Here's how the part is built. I have some questions about the finished solid (model axes, mm). A direction names the side the tool comes from. Round coordinates to 2 decimals unless told otherwise and drop trailing zeros. Loops run counter-clockwise (first coordinate to the right, second up) from the corner with the lowest first, then second, coordinate; pieces in that order, holes last. Notation, with made-up numbers: M 41.5,-1 L 64.5,-1 A15 cw 64.5,18 Z; hole C -22,31.5 d8. An arc over 180 degrees is marked long. Write each question's results on one line, items separated by ' | '. Start each with the question number.
```python
from build123d import *

# Parameters (mm, degrees)
SCHIZZO1_W                   = 94.84
SCHIZZO1_H                   = 59.15
ESTRUSIONE_ESTRUSIONE1_DEPTH = 0.8
SCHIZZO2_R                   = 1.5
TAGLIO_ESTRUSIONE1_DEPTH     = 56.909722097
SCHIZZO3_R                   = 0.445
TAGLIO_ESTRUSIONE2_DEPTH     = 56.909722097
ESTRUSIONE_ESTRUSIONE2_START = 0.01
SCHIZZO4_R                   = 2
SCHIZZO4_R_2                 = 1.5
SCHIZZO4_R_3                 = 0.745
SCHIZZO4_R_4                 = 0.445
ESTRUSIONE_ESTRUSIONE2_DEPTH = 0.01
SCHIZZO5_W                   = 85
SCHIZZO5_H                   = 55.26
ESTRUSIONE_ESTRUSIONE3_DEPTH = 2.4
SCHIZZO7_W                   = 73.44
SCHIZZO7_H                   = 48.96
TAGLIO_ESTRUSIONE3_DEPTH     = 0.5


with BuildPart() as part:
    # Schizzo1 → Estrusione-Estrusione1 (new, symmetric)
    with BuildSketch(Plane(origin=(0, 0, 0), x_dir=(1, 0, 0), z_dir=(0, 1, 0))):
        Rectangle(SCHIZZO1_W, SCHIZZO1_H)
    extrude(amount=ESTRUSIONE_ESTRUSIONE1_DEPTH, both=True)

    # Schizzo2 → Taglio-Estrusione1 (cut, through all)
    with BuildSketch(Plane(origin=(0, 0.8, 0), x_dir=(1, 0, 0), z_dir=(0, 1, 0))):
        with Locations(Location((-45.26, 24, 0), (0, 0, 270))):
            Circle(SCHIZZO2_R)
        with Locations(Location((44.75, 24, 0), (0, 0, 270))):
            Circle(SCHIZZO2_R)
        with Locations(Location((44.75, -24, 0), (0, 0, 270))):
            Circle(SCHIZZO2_R)
        with Locations(Location((-45.26, -24, 0), (0, 0, 270))):
            Circle(SCHIZZO2_R)
    extrude(amount=-TAGLIO_ESTRUSIONE1_DEPTH, mode=Mode.SUBTRACT)

    # Schizzo3 → Taglio-Estrusione2 (cut, through all)
    with BuildSketch(Plane(origin=(0, 0.8, 0), x_dir=(1, 0, 0), z_dir=(0, 1, 0))):
        with Locations(Location((-45.67, 0, 0), (0, 0, 270))):
            Circle(SCHIZZO3_R)
        with Locations(Location((-45.67, -2.54, 0), (0, 0, 270))):
            Circle(SCHIZZO3_R)
        with Locations(Location((-45.67, -5.08, 0), (0, 0, 270))):
            Circle(SCHIZZO3_R)
        with Locations(Location((-45.67, -7.62, 0), (0, 0, 270))):
            Circle(SCHIZZO3_R)
        with Locations(Location((-45.67, -10.16, 0), (0, 0, 270))):
            Circle(SCHIZZO3_R)
        with Locations(Location((-45.67, 2.54, 0), (0, 0, 270))):
            Circle(SCHIZZO3_R)
        with Locations(Location((-45.67, 5.08, 0), (0, 0, 270))):
            Circle(SCHIZZO3_R)
        with Locations(Location((-45.67, 7.62, 0), (0, 0, 270))):
            Circle(SCHIZZO3_R)
        with Locations(Location((-45.67, 10.16, 0), (0, 0, 270))):
            Circle(SCHIZZO3_R)
    extrude(amount=-TAGLIO_ESTRUSIONE2_DEPTH, mode=Mode.SUBTRACT)

    # Schizzo4 → Estrusione-Estrusione2 (add)
    # profile 1 of 13: a face of its own
    with BuildSketch(Plane(origin=(0, 0.8, 0), x_dir=(1, 0, 0), z_dir=(0, 1, 0)).offset(ESTRUSIONE_ESTRUSIONE2_START)):
        with Locations(Location((44.75, 24, 0), (0, 0, 90))):
            Circle(SCHIZZO4_R)
        with Locations(Location((44.75, 24, 0), (0, 0, 270))):
            Circle(SCHIZZO4_R_2, mode=Mode.SUBTRACT)
    # profile 2 of 13: a face of its own
    with BuildSketch(Plane(origin=(0, 0.8, 0), x_dir=(1, 0, 0), z_dir=(0, 1, 0)).offset(ESTRUSIONE_ESTRUSIONE2_START)):
        with Locations(Location((-45.26, 24, 0), (0, 0, 90))):
            Circle(SCHIZZO4_R)
        with Locations(Location((-45.26, 24, 0), (0, 0, 270))):
            Circle(SCHIZZO4_R_2, mode=Mode.SUBTRACT)
    # profile 3 of 13: a face of its own
    with BuildSketch(Plane(origin=(0, 0.8, 0), x_dir=(1, 0, 0), z_dir=(0, 1, 0)).offset(ESTRUSIONE_ESTRUSIONE2_START)):
        with Locations(Location((-45.26, -24, 0), (0, 0, 90))):
            Circle(SCHIZZO4_R)
        with Locations(Location((-45.26, -24, 0), (0, 0, 270))):
            Circle(SCHIZZO4_R_2, mode=Mode.SUBTRACT)
    # profile 4 of 13: a face of its own
    with BuildSketch(Plane(origin=(0, 0.8, 0), x_dir=(1, 0, 0), z_dir=(0, 1, 0)).offset(ESTRUSIONE_ESTRUSIONE2_START)):
        with Locations(Location((44.75, -24, 0), (0, 0, 90))):
            Circle(SCHIZZO4_R)
        with Locations(Location((44.75, -24, 0), (0, 0, 270))):
            Circle(SCHIZZO4_R_2, mode=Mode.SUBTRACT)
    # profile 5 of 13: a face of its own
    with BuildSketch(Plane(origin=(0, 0.8, 0), x_dir=(1, 0, 0), z_dir=(0, 1, 0)).offset(ESTRUSIONE_ESTRUSIONE2_START)):
        with Locations(Location((-45.67, 10.16, 0), (0, 0, 90))):
            Circle(SCHIZZO4_R_3)
        with Locations(Location((-45.67, 10.16, 0), (0, 0, 270))):
            Circle(SCHIZZO4_R_4, mode=Mode.SUBTRACT)
    # profile 6 of 13: a face of its own
    with BuildSketch(Plane(origin=(0, 0.8, 0), x_dir=(1, 0, 0), z_dir=(0, 1, 0)).offset(ESTRUSIONE_ESTRUSIONE2_START)):
        with Locations(Location((-45.67, 7.62, 0), (0, 0, 90))):
            Circle(SCHIZZO4_R_3)
        with Locations(Location((-45.67, 7.62, 0), (0, 0, 270))):
            Circle(SCHIZZO4_R_4, mode=Mode.SUBTRACT)
    # profile 7 of 13: a face of its own
    with BuildSketch(Plane(origin=(0, 0.8, 0), x_dir=(1, 0, 0), z_dir=(0, 1, 0)).offset(ESTRUSIONE_ESTRUSIONE2_START)):
        with Locations(Location((-45.67, 5.08, 0), (0, 0, 90))):
            Circle(SCHIZZO4_R_3)
        with Locations(Location((-45.67, 5.08, 0), (0, 0, 270))):
            Circle(SCHIZZO4_R_4, mode=Mode.SUBTRACT)
    # profile 8 of 13: a face of its own
    with BuildSketch(Plane(origin=(0, 0.8, 0), x_dir=(1, 0, 0), z_dir=(0, 1, 0)).offset(ESTRUSIONE_ESTRUSIONE2_START)):
        with Locations(Location((-45.67, 2.54, 0), (0, 0, 90))):
            Circle(SCHIZZO4_R_3)
        with Locations(Location((-45.67, 2.54, 0), (0, 0, 270))):
            Circle(SCHIZZO4_R_4, mode=Mode.SUBTRACT)
    # profile 9 of 13: a face of its own
    with BuildSketch(Plane(origin=(0, 0.8, 0), x_dir=(1, 0, 0), z_dir=(0, 1, 0)).offset(ESTRUSIONE_ESTRUSIONE2_START)):
        with Locations(Location((-45.67, 0, 0), (0, 0, 90))):
            Circle(SCHIZZO4_R_3)
        with Locations(Location((-45.67, 0, 0), (0, 0, 270))):
            Circle(SCHIZZO4_R_4, mode=Mode.SUBTRACT)
    # profile 10 of 13: a face of its own
    with BuildSketch(Plane(origin=(0, 0.8, 0), x_dir=(1, 0, 0), z_dir=(0, 1, 0)).offset(ESTRUSIONE_ESTRUSIONE2_START)):
        with Locations(Location((-45.67, -2.54, 0), (0, 0, 90))):
            Circle(SCHIZZO4_R_3)
        with Locations(Location((-45.67, -2.54, 0), (0, 0, 270))):
            Circle(SCHIZZO4_R_4, mode=Mode.SUBTRACT)
    # profile 11 of 13: a face of its own
    with BuildSketch(Plane(origin=(0, 0.8, 0), x_dir=(1, 0, 0), z_dir=(0, 1, 0)).offset(ESTRUSIONE_ESTRUSIONE2_START)):
        with Locations(Location((-45.67, -5.08, 0), (0, 0, 90))):
            Circle(SCHIZZO4_R_3)
        with Locations(Location((-45.67, -5.08, 0), (0, 0, 270))):
            Circle(SCHIZZO4_R_4, mode=Mode.SUBTRACT)
    # profile 12 of 13: a face of its own
    with BuildSketch(Plane(origin=(0, 0.8, 0), x_dir=(1, 0, 0), z_dir=(0, 1, 0)).offset(ESTRUSIONE_ESTRUSIONE2_START)):
        with Locations(Location((-45.67, -7.62, 0), (0, 0, 90))):
            Circle(SCHIZZO4_R_3)
        with Locations(Location((-45.67, -7.62, 0), (0, 0, 270))):
            Circle(SCHIZZO4_R_4, mode=Mode.SUBTRACT)
    # profile 13 of 13: a face of its own
    with BuildSketch(Plane(origin=(0, 0.8, 0), x_dir=(1, 0, 0), z_dir=(0, 1, 0)).offset(ESTRUSIONE_ESTRUSIONE2_START)):
        with Locations(Location((-45.67, -10.16, 0), (0, 0, 90))):
            Circle(SCHIZZO4_R_3)
        with Locations(Location((-45.67, -10.16, 0), (0, 0, 270))):
            Circle(SCHIZZO4_R_4, mode=Mode.SUBTRACT)
    estrusione_estrusione2 = extrude(amount=-ESTRUSIONE_ESTRUSIONE2_DEPTH)

    # Specchia1: Estrusione-Estrusione2 across plane
    add(estrusione_estrusione2.mirror(Plane.ZX))

    # Schizzo5 → Estrusione-Estrusione3 (add)
    with BuildSketch(Plane(origin=(0, 0.8, 0), x_dir=(1, 0, 0), z_dir=(0, 1, 0))):
        with Locations((-0.02, 0)):
            Rectangle(SCHIZZO5_W, SCHIZZO5_H)
    extrude(amount=ESTRUSIONE_ESTRUSIONE3_DEPTH)

    # Schizzo7 → Taglio-Estrusione3 (cut)
    with BuildSketch(Plane(origin=(0, 3.2, 0), x_dir=(1, 0, 0), z_dir=(0, 1, 0))):
        with Locations((-3.05, 0)):
            Rectangle(SCHIZZO7_W, SCHIZZO7_H)
    extrude(amount=-TAGLIO_ESTRUSIONE3_DEPTH, mode=Mode.SUBTRACT)


solid = part.part
```
Item 1: Which directions (+Z, -Z, +X, -X, +Y, -Y) give clear straight access to the entire face, cutting with the end or side of a thin tool? Please do faces 4 (the face through (-1, 2, 27.63)), 5 (the face through (-1, -0.8, 0)), 6 (the face through (43, 0.81, -24)), 7 (the face through (-47, 0.81, -24)).
Item 2: If we mould it in two halves opening along X, with no side actions, what happens to faces 1 (the face through (42.48, 2, 0)), 2 (the face through (-47, -0.81, -24)), 3 (the face through (-4, 2.7, 0))? For each: released by +X, released by -X, zero draft, split by the parting line, or undercut.
Item 3: If we section it at C-C on z = 20.5: Please give me the cut outline in (x, y).
Item 4: If we section it at D-D on y = 1.9: Please give me the cut outline in (x, z).
Item 5: I need wall thicknesses on L1, parallel to X at y = 0, z = 24; L2, parallel to X at y = 2.9, z = 7; L3, parallel to Z at x = 8, y = 1.95. Which ranges of each line are inside material? Lowest first, please.
Item 6: I'm going to push flat-ended pins straight in: pin 1 (3 mm diameter, centred on x = -46, z = -23, fed in from +Y); pin 2 (2.5 mm diameter, centred on x = -45.26, z = 24, fed in from +Y); pin 3 (10 mm diameter, centred on x = 7.5, z = 11.5, fed in from -Y); pin 4 (0.6 mm diameter, centred on x = 13.5, y = 3, fed in from +Z). Where does each tip first touch, or does it pass through?
Item 7: If we section it at A-A on x = 44.75: Please give me the cut outline in (y, z) (3 decimals), and give its area (3 significant figures).
Item 8: If we section it at B-B on x = -24.5: Please give me the cut outline in (y, z) (3 decimals), and give its area (3 significant figures).
Numbers:
1) face 4: +Z, +X, -X, +Y | face 5: +Z, -Z, +X, -X, -Y | face 6: +Z, -Z, +X, +Y | face 7: +Z, -Z, -X, +Y
2) face 1: released by +X | face 2: zero draft | face 3: undercut
3) outline: M -47.42,-0.8 L 47.42,-0.8 L 47.42,0.8 L 42.48,0.8 L 42.48,3.2 L 33.67,3.2 L 33.67,2.7 L -39.77,2.7 L -39.77,3.2 L -42.52,3.2 L -42.52,0.8 L -47.42,0.8 Z
4) outline: M -42.52,-27.63 L 42.48,-27.63 L 42.48,27.63 L -42.52,27.63 Z
5) L1: -47.42 to -46.76, -43.76 to 43.25, 46.25 to 47.42 | L2: -42.52 to -39.77, 33.67 to 42.48 | L3: -27.63 to 27.63
6) pin 1: y = 0.81 | pin 2: through | pin 3: y = -0.8 | pin 4: z = 27.63
7) outline: M -0.81,-26 L -0.8,-26 L -0.8,-29.575 L 0.8,-29.575 L 0.8,-26 L 0.81,-26 L 0.81,-25.5 L -0.81,-25.5 Z; M -0.81,-22.5 L 0.81,-22.5 L 0.81,-22 L 0.8,-22 L 0.8,22 L 0.81,22 L 0.81,22.5 L -0.81,22.5 L -0.81,22 L -0.8,22 L -0.8,-22 L -0.81,-22 Z; M -0.81,25.5 L 0.81,25.5 L 0.81,26 L 0.8,26 L 0.8,29.575 L -0.8,29.575 L -0.8,26 L -0.81,26 Z | area: 85.1 mm²
8) outline: M -0.8,-29.575 L 0.8,-29.575 L 0.8,-27.63 L 3.2,-27.63 L 3.2,-24.48 L 2.7,-24.48 L 2.7,24.48 L 3.2,24.48 L 3.2,27.63 L 0.8,27.63 L 0.8,29.575 L -0.8,29.575 Z | area: 203 mm²
